Check sheet for the modelled part. Datum: model origin and axes. Units: mm. A direction names the side the tool comes from. Give positions to 0.01 mm unless a question says otherwise; leave off trailing zeros. Loops run counter-clockwise (first coordinate to the right, second up) from the corner with the lowest first, then second, coordinate; pieces in that order, holes last. Notation, with made-up numbers: (75.25, -33) - (95.25, -33) arc R23 cw to (95.25, 4) - close; hole circle Ø5 at (52.25, -1.5). An arc over 180 degrees is marked (long way). Use one line per item in the form item = value.
from build123d import *

# Parameters (mm, degrees)
SKETCH1_R           = 5
BOSS_EXTRUDE1_DEPTH = 10


with BuildPart() as part:
    # Sketch1 → Boss-Extrude1 (new body)
    with BuildSketch(Plane.XY):
        Polygon((-35, 30), (-25, 40), (25, 40), (35, 30), (35, 0), (25, 0), (25, 10), (15, 10), (15, 0), (-15, 0), (-15, 10), (-25, 10), (-25, 0), (-35, 0), align=None)
        with Locations((-25, 30)):
            Circle(SKETCH1_R, mode=Mode.SUBTRACT)
        with Locations((25, 30)):
            Circle(SKETCH1_R, mode=Mode.SUBTRACT)
        Polygon((15, 15), (-15, 15), (-15, 25), (-5, 25), (-5, 20), (5, 20), (5, 25), (15, 25), align=None, mode=Mode.SUBTRACT)
    extrude(amount=BOSS_EXTRUDE1_DEPTH)


solid = part.part
Item 1: Section check B-B on x = -3.5. Record the boundary of the cut face in (y, z), then the cut area to 3 significant figures.
Answer block:
outline = (0, 0) - (15, 0) - (15, 10) - (0, 10) - close; (20, 0) - (40, 0) - (40, 10) - (20, 10) - close
area = 350 mm2
Item 2: Access from +Z, -Z, +X, -X, +Y, -Y to the whole of each face (thin tool, end or side, straight path). Record for faces 4 (the face through (-35, 15, 5)), 5 (the face through (-15, 20, 5)), 6 (the face through (20, 10, 5)).
Answer block:
face_4 = +Z, -Z, -X, +Y, -Y
face_5 = +Z, -Z
face_6 = +Z, -Z, -Y
Item 3: Section check A-A on y = 16. Record the boundary of the cut face in (x, z).
Answer block:
outline = (-35, 0) - (-15, 0) - (-15, 10) - (-35, 10) - close; (15, 0) - (35, 0) - (35, 10) - (15, 10) - close
Item 4: Thickness scan on L1, parallel to X at y = 8, z = 9; L2, parallel to Y at x = 2, z = 8.25; L3, parallel to X at y = 26, z = 7.25. Record the ranges inside material, lowest first.
Answer block:
L1 = -35 to -25, -15 to 15, 25 to 35
L2 = 0 to 15, 20 to 40
L3 = -35 to -28, -22 to 22, 28 to 35
Item 5: Section check C-C on y = 4. Record the boundary of the cut face in (x, z), then the cut area to 3 significant figures.
Answer block:
outline = (-35, 0) - (-25, 0) - (-25, 10) - (-35, 10) - close; (-15, 0) - (15, 0) - (15, 10) - (-15, 10) - close; (25, 0) - (35, 0) - (35, 10) - (25, 10) - close
area = 500 mm2
Item 6: Mould release check, pull along X, two halves, no side actions. Record for faces 1 (the face through (30, 0, 5)), 2 (the face through (0, 20, 5)), 3 (the face through (-30, 35, 5)): released by +X, released by -X, zero draft, split by the parting line, or undercut.
Answer block:
face_1 = zero draft
face_2 = undercut
face_3 = released by -X
Item 7: Section check D-D on z = 3.5. Record the boundary of the cut face in (x, y), then the cut area to 3 significant figures.
Answer block:
outline = (-35, 0) - (-25, 0) - (-25, 10) - (-15, 10) - (-15, 0) - (15, 0) - (15, 10) - (25, 10) - (25, 0) - (35, 0) - (35, 30) - (25, 40) - (-25, 40) - (-35, 30) - close; hole circle Ø10 at (-25, 30); hole (-15, 15) - (15, 15) - (15, 25) - (5, 25) - (5, 20) - (-5, 20) - (-5, 25) - (-15, 25) - close; hole circle Ø10 at (25, 30)
area = 2,090 mm2
